```python
from build123d import *

# Parameters (mm, degrees)
F0_R      = 12.7
F1_DEPTH  = 127
F2_R      = 7.9375
F3_DEPTH  = 88.899746
F6_DEPTH  = 40.64
F8_R      = 9.525
F9_DEPTH  = 15.24
F10_D     = 12.7
F10_DEPTH = 11.43
F10_TIP   = 3.8154649308
F4_R      = 4.7625
F11_DEPTH = 50.8
F12_R     = 6.35
F13_DEPTH = 11.43


with BuildPart() as f1:
    # F0 (on Top) → F1 (new body)
    with BuildSketch(Plane.XY):
        Circle(F0_R)
    extrude(amount=F1_DEPTH)

    # F2 (on face) → F3 (cut)
    with BuildSketch(Plane.XY.offset(127)):
        Circle(F2_R)
    extrude(amount=-F3_DEPTH, mode=Mode.SUBTRACT)

    # F5 (on face) → F6 (cut)
    with BuildSketch(Plane(origin=(0, 0, 0), x_dir=(1, 0, 0), z_dir=(0, 0, -1))):
        with BuildLine():
            Line((6.6901401331, -10.795), (-6.6901401331, -10.795))
            ThreePointArc((-6.6901401331, -10.795), (0, -12.7), (6.6901401331, -10.795))
        make_face()
    extrude(amount=-F6_DEPTH, mode=Mode.SUBTRACT)

    # F8 (on face) → F9 (cut)
    with BuildSketch(Plane.XY.offset(127)):
        Circle(F8_R)
    extrude(amount=-F9_DEPTH, mode=Mode.SUBTRACT)

    # F10
    with Locations(Plane(origin=(0, 10.795, 0), x_dir=(-1, 0, 0), z_dir=(0, 1, 0))):
        with Locations((0, 31.75)):
            Hole(F10_D / 2, depth=F10_DEPTH)
            with Locations((0, 0, -(F10_DEPTH + F10_TIP / 2))):  # 118° drill point
                Cone(0, F10_D / 2, F10_TIP, mode=Mode.SUBTRACT)

    # F4 (on face) → F11 (cut)
    with BuildSketch(Plane(origin=(0, 0, 0), x_dir=(1, 0, 0), z_dir=(0, 0, -1))):
        with Locations((0, 0.1964742664)):
            Circle(F4_R)
    extrude(amount=-F11_DEPTH, mode=Mode.SUBTRACT)

    # F12 (on Top) → F13 (cut)
    with BuildSketch(Plane.XY):
        Circle(F12_R)
    extrude(amount=F13_DEPTH, mode=Mode.SUBTRACT)


solid = f1.part
```
Verification items for the finished model (mm, model axes). A direction names the side the tool comes from. Round coordinates to 2 decimals unless told otherwise and drop trailing zeros. Write each loop counter-clockwise with the first axis right and the second up, starting at its lowest first coordinate (ties: lowest second). Pieces come first, ordered by that corner, then holes.
1. Section check D-D on z = 109.5. Enter the section's corners in (x, y) (1 decimal).
2. Access from +Z, -Z, +X, -X, +Y, -Y to the whole of each face (thin tool, end or side, straight path). Record for faces 4 (the cylindrical face through (-5.04, 6.27, 27.89)), 5 (the cylindrical face through (-7.559, -5.796, 119.487)), 6 (the flat face through (-1, 5, 11.43)), 7 (the flat face through (0, 10.795, 16)).
3. Section check A-A on x = 0. State how many separate pieces and enclosed holes the cut face has, plus the area to 3 significant figures.
4. Draft check along X on faces 1 (the cylindrical face through (-2.75, -12.4, 62.61)), 2 (the flat face through (3, -6, 0)), 3 (the flat face through (3, 4, 38.1)). Enter one of: +X half, -X half, draft (parallel to the pull), parting line (faces both ways), or undercut.
5. Section check C-C on y = 2.75. Enter the section's corners in (x, z).
6. Scan lines: L1, parallel to Y at x = 0, z = 6 (3 decimals); L2, parallel to Y at x = 0, z = 27; L3, parallel to Y at x = 0, z = 76.5. Record each from-to range of solid material in increasing order.
7. Gauge pin test, flat ends, axial feed: P1, Ø14.5, axis at x = 0, y = 0, coming from the +Z side; P2, Ø8, axis at x = 10, y = 6.5, coming from the -Z side; P3, Ø11.5, axis at x = 0, y = 0, coming from the -Z side; P4, Ø0.6, axis at x = 3, y = 12, coming from the -Z side. Record the tip position at first contact, or that the pin passes through.
Answer:
1. outline: circle Ø25.4 at (0, 0); hole circle Ø15.9 at (0, 0)
2. face 4: +Y
2. face 5: +Z
2. face 6: -Z
2. face 7: -Z, +X, -X, +Y
3. separate pieces: 3
3. enclosed holes: 0
3. area: 1,210 mm2
4. face 1: parting line
4. face 2: draft
4. face 3: undercut
5. outline: (-12.4, 0) - (-5.72, 0) - (-5.72, 11.43) - (-3.74, 11.43) - (-3.74, 26.62) arc R6.35 cw to (-3.74, 36.88) - (-3.74, 38.1) - (-7.45, 38.1) - (-7.45, 111.76) - (-9.12, 111.76) - (-9.12, 127) - (-12.4, 127) - close; (3.74, 11.43) - (5.72, 11.43) - (5.72, 0) - (12.4, 0) - (12.4, 127) - (9.12, 127) - (9.12, 111.76) - (7.45, 111.76) - (7.45, 38.1) - (3.74, 38.1) - (3.74, 36.88) arc R6.35 cw to (3.74, 26.62) - close
6. L1: y = -12.7 to -6.35, 6.35 to 10.795
6. L2: y = -12.7 to -4.96
6. L3: y = -12.7 to -7.94, 7.94 to 12.7
7. P1: stops at z = 38.1
7. P2: stops at z = 0
7. P3: stops at z = 11.43
7. P4: stops at z = 40.64
